```python
from build123d import *

# Parameters (mm, degrees)
SKETCH3_W           = 190
SKETCH3_H           = 80
BOSS_EXTRUDE1_DEPTH = 5
SKETCH4_R           = 1.5
CUT_EXTRUDE1_DEPTH  = 5
SKETCH5_R           = 3
SKETCH5_R_2         = 1.5
CUT_EXTRUDE2_DEPTH  = 2
FILLET1_R           = 0.5


with BuildPart() as part:
    # Sketch3 → Boss-Extrude1 (new body)
    with BuildSketch(Plane(origin=(0, 0, 0), x_dir=(1, 0, 0), z_dir=(0, 1, 0))):
        Rectangle(SKETCH3_W, SKETCH3_H)
    extrude(amount=BOSS_EXTRUDE1_DEPTH)

    # Sketch4 → Cut-Extrude1 (cut)
    with BuildSketch(Plane(origin=(0, 5, 0), x_dir=(1, 0, 0), z_dir=(0, 1, 0))):
        with Locations(Location((-92.5, 35, 0), (0, 0, 270))):
            Circle(SKETCH4_R)
        with Locations(Location((-92.5, 25, 0), (0, 0, 270))):
            Circle(SKETCH4_R)
        with Locations(Location((-92.5, 15, 0), (0, 0, 270))):
            Circle(SKETCH4_R)
        with Locations(Location((-92.5, 5, 0), (0, 0, 270))):
            Circle(SKETCH4_R)
        with Locations(Location((-92.5, -5, 0), (0, 0, 270))):
            Circle(SKETCH4_R)
        with Locations(Location((-92.5, -15, 0), (0, 0, 270))):
            Circle(SKETCH4_R)
        with Locations(Location((-92.5, -25, 0), (0, 0, 270))):
            Circle(SKETCH4_R)
        with Locations(Location((-92.5, -35, 0), (0, 0, 270))):
            Circle(SKETCH4_R)
        with Locations(Location((92.5, -35, 0), (0, 0, 90))):
            Circle(SKETCH4_R)
        with Locations(Location((92.5, -25, 0), (0, 0, 90))):
            Circle(SKETCH4_R)
        with Locations(Location((92.5, -15, 0), (0, 0, 90))):
            Circle(SKETCH4_R)
        with Locations(Location((92.5, -5, 0), (0, 0, 90))):
            Circle(SKETCH4_R)
        with Locations(Location((92.5, 5, 0), (0, 0, 90))):
            Circle(SKETCH4_R)
        with Locations(Location((92.5, 15, 0), (0, 0, 90))):
            Circle(SKETCH4_R)
        with Locations(Location((92.5, 35, 0), (0, 0, 90))):
            Circle(SKETCH4_R)
        with Locations(Location((92.5, 25, 0), (0, 0, 90))):
            Circle(SKETCH4_R)
    extrude(amount=-CUT_EXTRUDE1_DEPTH, mode=Mode.SUBTRACT)

    # Sketch5 → Cut-Extrude2 (cut)
    # profile 1 of 16: a face of its own
    with BuildSketch(Plane(origin=(0, 5, 0), x_dir=(1, 0, 0), z_dir=(0, 1, 0))):
        with Locations((-92.5, 35)):
            Circle(SKETCH5_R)
        with Locations(Location((-92.5, 35, 0), (0, 0, 270))):
            Circle(SKETCH5_R_2, mode=Mode.SUBTRACT)
    # profile 2 of 16: a face of its own
    with BuildSketch(Plane(origin=(0, 5, 0), x_dir=(1, 0, 0), z_dir=(0, 1, 0))):
        with Locations((92.5, 35)):
            Circle(SKETCH5_R)
        with Locations(Location((92.5, 35, 0), (0, 0, 270))):
            Circle(SKETCH5_R_2, mode=Mode.SUBTRACT)
    # profile 3 of 16: a face of its own
    with BuildSketch(Plane(origin=(0, 5, 0), x_dir=(1, 0, 0), z_dir=(0, 1, 0))):
        with Locations((-92.5, 25)):
            Circle(SKETCH5_R)
    # profile 4 of 16: a face of its own
    with BuildSketch(Plane(origin=(0, 5, 0), x_dir=(1, 0, 0), z_dir=(0, 1, 0))):
        with Locations((92.5, 25)):
            Circle(SKETCH5_R)
    # profile 5 of 16: a face of its own
    with BuildSketch(Plane(origin=(0, 5, 0), x_dir=(1, 0, 0), z_dir=(0, 1, 0))):
        with Locations((-92.5, 15)):
            Circle(SKETCH5_R)
    # profile 6 of 16: a face of its own
    with BuildSketch(Plane(origin=(0, 5, 0), x_dir=(1, 0, 0), z_dir=(0, 1, 0))):
        with Locations((92.5, 15)):
            Circle(SKETCH5_R)
    # profile 7 of 16: a face of its own
    with BuildSketch(Plane(origin=(0, 5, 0), x_dir=(1, 0, 0), z_dir=(0, 1, 0))):
        with Locations((-92.5, 5)):
            Circle(SKETCH5_R)
    # profile 8 of 16: a face of its own
    with BuildSketch(Plane(origin=(0, 5, 0), x_dir=(1, 0, 0), z_dir=(0, 1, 0))):
        with Locations((92.5, 5)):
            Circle(SKETCH5_R)
    # profile 9 of 16: a face of its own
    with BuildSketch(Plane(origin=(0, 5, 0), x_dir=(1, 0, 0), z_dir=(0, 1, 0))):
        with Locations((-92.5, -5)):
            Circle(SKETCH5_R)
    # profile 10 of 16: a face of its own
    with BuildSketch(Plane(origin=(0, 5, 0), x_dir=(1, 0, 0), z_dir=(0, 1, 0))):
        with Locations((92.5, -5)):
            Circle(SKETCH5_R)
    # profile 11 of 16: a face of its own
    with BuildSketch(Plane(origin=(0, 5, 0), x_dir=(1, 0, 0), z_dir=(0, 1, 0))):
        with Locations((-92.5, -15)):
            Circle(SKETCH5_R)
    # profile 12 of 16: a face of its own
    with BuildSketch(Plane(origin=(0, 5, 0), x_dir=(1, 0, 0), z_dir=(0, 1, 0))):
        with Locations((92.5, -15)):
            Circle(SKETCH5_R)
    # profile 13 of 16: a face of its own
    with BuildSketch(Plane(origin=(0, 5, 0), x_dir=(1, 0, 0), z_dir=(0, 1, 0))):
        with Locations((-92.5, -25)):
            Circle(SKETCH5_R)
    # profile 14 of 16: a face of its own
    with BuildSketch(Plane(origin=(0, 5, 0), x_dir=(1, 0, 0), z_dir=(0, 1, 0))):
        with Locations((92.5, -25)):
            Circle(SKETCH5_R)
    # profile 15 of 16: a face of its own
    with BuildSketch(Plane(origin=(0, 5, 0), x_dir=(1, 0, 0), z_dir=(0, 1, 0))):
        with Locations((-92.5, -35)):
            Circle(SKETCH5_R)
    # profile 16 of 16: a face of its own
    with BuildSketch(Plane(origin=(0, 5, 0), x_dir=(1, 0, 0), z_dir=(0, 1, 0))):
        with Locations((92.5, -35)):
            Circle(SKETCH5_R)
    extrude(amount=-CUT_EXTRUDE2_DEPTH, mode=Mode.SUBTRACT)

    # Fillet1
    fillet1_edges = [part.edges().sort_by_distance(p)[0] for p in [
        (-95, 4, -33.341687605),
        (-95, 4, -36.658312395),
        (-95, 4, 26.658312395),
        (-95, 4, 23.341687605),
        (-95, 4, 16.658312395),
        (-95, 4, 13.341687605),
        (-95, 4, 36.658312395),
        (-95, 4, 33.341687605),
        (-95, 4, -13.341687605),
        (-95, 4, -16.658312395),
        (-95, 4, -23.341687605),
        (-95, 4, -26.658312395),
        (-95, 4, 6.658312395),
        (-95, 4, 3.341687605),
        (-95, 4, -3.341687605),
        (-95, 4, -6.658312395),
        (95, 4, 13.341687605),
        (95, 4, 16.658312395),
        (95, 4, 3.341687605),
        (95, 4, 6.658312395),
        (95, 4, 33.341687605),
        (95, 4, 36.658312395),
        (95, 4, 23.341687605),
        (95, 4, 26.658312395),
        (95, 4, -26.658312395),
        (95, 4, -23.341687605),
        (95, 4, -36.658312395),
        (95, 4, -33.341687605),
        (95, 4, -6.658312395),
        (95, 4, -3.341687605),
        (95, 4, -16.658312395),
        (95, 4, -13.341687605),
    ]]
    fillet(fillet1_edges, radius=FILLET1_R)


solid = part.part
```
Verification items for the finished model (mm, model axes). Coordinates: 2 decimals unless noted, no trailing zeros. Put each result on its own line as item: value. Start each with the question number.
1) Material ranges on L1, parallel to X at y = 0.9, z = 15; L2, parallel to X at y = 2.9, z = -6; L3, parallel to X at y = 3.75, z = 25, recorded low to high.
2) Go/stop test with flat-tipped pins: pin 1 (5 mm diameter, centred on x = -92.5, z = 35, fed in from +Y); pin 2 (7 mm diameter, centred on x = -92.5, z = 25, fed in from -Y). Record where each tip stops, or that it passes through.
3) Release check for a two-part mould opening along Z. For faces 1 (the flat face through (91, 3, -6)), 2 (the flat face through (-1, 2, -40)), 3 (the flat face through (-1, 5, -1)) record: pulls with the +Z half, pulls with the -Z half, needs draft (parallel to the pull), parting line crosses it, or undercut.
Geometry check:
1. L1: x = -95 to -94, -91 to 91, 94 to 95
1. L2: x = -95 to -93.62, -91.38 to 91.38, 93.62 to 95
1. L3: x = -89.5 to 89.5
2. pin 1: stops at y = 3
2. pin 2: stops at y = 0
3. face 1: undercut
3. face 2: pulls with the -Z half
3. face 3: needs draft
